```python
from build123d import *

# Parameters (mm, degrees)
F0_W     = 32
F0_H     = 10
F1_DEPTH = 16.6
F2_R     = 5
F3_R     = 4.99999
F4_R     = 4.99999


# Not quite as in the source:
# - a fillet or chamfer is up to 0.001 mm smaller than in the source, because OpenCascade refuses the exact size


with BuildPart() as f1:
    # F0 (on Front) → F1 (new body)
    with BuildSketch(Plane.XZ):
        Rectangle(F0_W, F0_H)
    extrude(amount=F1_DEPTH)

    # F2
    f2_edges = [f1.edges().sort_by_distance(p)[0] for p in [
        (16, -8.3, 5),
    ]]
    fillet(f2_edges, radius=F2_R)

    # F3 (radius 5 in the source; OpenCascade refuses exactly that, so slightly less here)
    f3_edges = [f1.edges().sort_by_distance(p)[0] for p in [
        (-16, -8.3, 5),
        (16, -8.3, -5),
        (-16, -8.3, -5),
    ]]
    fillet(f3_edges, radius=F3_R)

    # F4 (radius 5 in the source; OpenCascade refuses exactly that, so slightly less here)
    f4_edges = [f1.edges().sort_by_distance(p)[0] for p in [
        (-5e-06, -16.6, 5),
    ]]
    fillet(f4_edges, radius=F4_R)


solid = f1.part
```
CAD build for the part. Positions are in the model's coordinates, mm. Coordinates: 2 decimals unless noted, no trailing zeros. Order: outer loops, then holes, each group sorted by start corner. A loop starts at its lowest first (then second) coordinate and runs counter-clockwise, first axis right, second up. Notation, with made-up numbers: (39, 75) - (55, 75) arc R27 cw to (55, 104) - close; hole circle Ø7 at (69.5, -18.75). An arc over 180 degrees is marked (long way). Use a Markdown table: item, result. Add a question column.
(1) Saw through at C-C (z = -0.5). Give the cut face in (x, y), then the cut area to 3 significant figures.
(2) Drill centre lines: line 1 along Y through (x, z) = (-5.5, 0.25); line 2 along Z through (x, y) = (-1, -11.75); line 3 along Y through (x, z) = (-8, 1). Where is each one in solid material? Low to high. Write a range as [from, to].
(3) Flat gauge pin, fed straight in: pin 1 (1 mm diameter, centred on x = 1.5, z = 1, fed in from -Y). Where does the tip first touch, or does it go through?
Solved:
| question | item | result |
|---|---|---|
| 1 | outline | (-15.97, -11.6) arc R4.97 ccw to (-11, -16.57) - (11, -16.57) arc R4.97 ccw to (15.97, -11.6) - (15.97, 0) - (-15.97, 0) - close |
| 1 | area | 519 mm² |
| 2 | line 1 | y = [-16.59, 0] |
| 2 | line 2 | z = [-5, 5] |
| 2 | line 3 | y = [-16.5, 0] |
| 3 | pin 1 | stops at y = -16.57 |
